Source: CAD feature listing. Evaluate the final solid. Frame: model axes, mm. A direction names the side the tool comes from. Give positions to 0.01 mm unless a question says otherwise; leave off trailing zeros. Write each loop counter-clockwise with the first axis right and the second up, starting at its lowest first coordinate (ties: lowest second). Pieces come first, ordered by that corner, then holes. Notation, with made-up numbers: (2, 45.5) -> (29, 45.5) arc R5 ccw to (29, 52.5) -> close; hole circle Ø6 at (-40, 72.25). An arc over 180 degrees is marked (long way). Use a Markdown table: item, result. Add a question column.
```python
from build123d import *

# Parameters (mm, degrees)
F0_W      = 29
F0_H      = 16.5
F1_DEPTH  = 38.5
F2_T      = -2
F3_DEPTH  = 2.25
F4_SIZE   = 2
F5_SIZE   = 0.99999
F7_DEPTH  = 16.501
F9_DEPTH  = 2
F10_R     = 2
F11_DEPTH = 2.001
F12_W     = 5.538
F12_H     = 5.533
F14_W     = 5.538
F14_H     = 4.583


# Not quite as in the source:
# - a fillet or chamfer is up to 0.001 mm smaller than in the source, because OpenCascade refuses the exact size


with BuildPart() as f1:
    # F0 (on Top) → F1 (new body)
    with BuildSketch(Plane.XY):
        with Locations((14.5, 8.25)):
            Rectangle(F0_W, F0_H)
    extrude(amount=F1_DEPTH)

    # F2
    f2_openings = [f1.faces().sort_by_distance(p)[0] for p in [
        (14.5, 8.25, 38.5),
    ]]
    offset(amount=F2_T, openings=f2_openings)

    # F3 (add): a face of the model
    f3_faces = [f1.faces().sort_by_distance(p)[0] for p in [
        (14.5, 8.25, 2),
    ]]
    extrude(f3_faces, amount=F3_DEPTH)

    # F4
    f4_edges = [f1.edges().sort_by_distance(p)[0] for p in [
        (29, 0, 19.25),
        (29, 16.5, 19.25),
        (0, 0, 19.25),
        (0, 16.5, 19.25),
        (14.5, 0, 0),
        (0, 8.25, 0),
        (14.5, 16.5, 0),
        (29, 8.25, 0),
    ]]
    chamfer(f4_edges, length=F4_SIZE)

    # F5 (size 1 in the source; OpenCascade refuses exactly that, so slightly less here)
    f5_edges = [f1.edges().sort_by_distance(p)[0] for p in [
        (14.5, 0, 38.5),
        (29, 8.25, 38.5),
        (14.5, 16.5, 38.5),
        (0, 8.25, 38.5),
    ]]
    chamfer(f5_edges, length=F5_SIZE)

    # F6 (on face) → F7 (cut, through all)
    with BuildSketch(Plane.XZ):
        Polygon((6.464, 8.664), (6.464, 4.94), (23.536, 4.94), (23.536, 8.664), (17.364, 12.834), (12.635, 12.834), align=None)
    extrude(amount=-F7_DEPTH, mode=Mode.SUBTRACT)

    # F8 (on Right) → F9 (cut, through all)
    with BuildSketch(Plane.YZ):
        with BuildLine():
            Line((14.5, 38.5), (2, 38.5))
            Line((2, 38.5), (2, 28.5))
            ThreePointArc((2, 28.5), (8.25, 34.75), (14.5, 28.5))
            Line((14.5, 28.5), (14.5, 38.5))
        make_face()
        with BuildLine():
            ThreePointArc((14.5, 28.5), (8.25, 34.75), (2, 28.5))
            Line((2, 28.5), (14.5, 28.5))
        make_face()
        with BuildLine():
            Line((14.5, 28.5), (2, 28.5))
            ThreePointArc((2, 28.5), (2.8042583777, 25.4330148055), (5.0100474186, 23.1553571429))
            ThreePointArc((5.0100474186, 23.1553571429), (8.25, 26.15), (11.4899525814, 23.1553571429))
            ThreePointArc((11.4899525814, 23.1553571429), (13.6957416223, 25.4330148055), (14.5, 28.5))
        make_face()
        with BuildLine():
            ThreePointArc((11.4899525814, 23.1553571429), (8.25, 26.15), (5.0100474186, 23.1553571429))
            ThreePointArc((5.0100474186, 23.1553571429), (8.25, 22.25), (11.4899525814, 23.1553571429))
        make_face()
        with BuildLine():
            ThreePointArc((11.4899525814, 23.1553571429), (8.25, 22.25), (5.0100474186, 23.1553571429))
            ThreePointArc((5.0100474186, 23.1553571429), (8.122222634, 19.6525128261), (11.5, 22.9))
            ThreePointArc((11.5, 22.9), (11.4974871739, 23.027777366), (11.4899525814, 23.1553571429))
        make_face()
    extrude(amount=F9_DEPTH, mode=Mode.SUBTRACT)

    # F10 (on face) → F11 (cut, through all)
    with BuildSketch(Plane(origin=(27, 0, 0), x_dir=(0, -1, 0), z_dir=(-1, 0, 0))):
        with Locations((-8.25, 22.9)):
            Circle(F10_R)
    extrude(amount=-F11_DEPTH, mode=Mode.SUBTRACT)

    # F12 (on face) → F15 section 0
    with BuildSketch(Plane(origin=(0, 0, 0), x_dir=(0, -1, 0), z_dir=(-1, 0, 0))):
        with Locations((-8.25, 8.0385)):
            Rectangle(F12_W, F12_H)
    # F14 (on offset) → F15 section 1
    with BuildSketch(Plane(origin=(4.45, 0, 0), x_dir=(0, -1, 0), z_dir=(-1, 0, 0))):
        with Locations((-8.25, 8.5135)):
            Rectangle(F14_W, F14_H)
    loft(mode=Mode.SUBTRACT)


solid = f1.part
```
(1) Access query for faces 1 (the flat face through (15, 15, 4.94)), 2 (the flat face through (2, 8, 14)), 3 (the flat face through (1.4, 1.4, 1.2)), 4 (the flat face through (1, 8, 10.805)). Directions: +Z, -Z, +X, -X, +Y, -Y. A direction counts if a zero-diameter tool reaches every point of the face in a straight line with its end or side. Return the directions, or none.
(2) Mould query, pull axis Y, two halves, no side actions, for faces 5 (the flat face through (20.49, 0.99, 10.72)), 6 (the flat face through (14, 8, 4.25)), 7 (the flat face through (14, 16, 38)), 8 (the flat face through (14, 1, 1)). Classes: +Y half, -Y half, draft (parallel to the pull), parting line (faces both ways), or undercut.
(3) First-contact query: pin 1 Ø1.5 at (x, y) = (21.5, 12.5) entering from +Z; pin 2 Ø1 at (y, z) = (1, 6.5) entering from +X; pin 3 Ø0.6 at (x, y) = (0.5, 7) entering from -Z. Flat tips, straight axial feed; report the tip coordinate or a pass-through.
(4) Cut plane A-A on x = 16. Return the cut outline in (y, z).
(5) Cut plane C-C on y = 13.25. Return the cut outline in (x, z).
(6) Material intervals for L1, parallel to Y at x = 25, z = 9; L2, parallel to X at y = 12.25, z = 4.5; L3, parallel to Z at x = 17, y = 14, sorted ascending.
(7) Cut plane B-B on z = 16. Return the cut outline in (x, y).
(8) Cut plane D-D on y = 8.25. Return the cut outline in (x, z) (3 decimals).
Output:
| question | item | result |
|---|---|---|
| 1 | face 1 | +Y, -Y |
| 1 | face 2 | +Z |
| 1 | face 3 | -Z, -X, -Y |
| 1 | face 4 | -X |
| 2 | face 5 | draft |
| 2 | face 6 | undercut |
| 2 | face 7 | +Y half |
| 2 | face 8 | -Y half |
| 3 | pin 1 | z = 4.25 |
| 3 | pin 2 | x = 28.5 |
| 3 | pin 3 | z = 1.2 |
| 4 | outline | (0, 2) -> (2, 0) -> (14.5, 0) -> (16.5, 2) -> (16.5, 4.94) -> (14.5, 4.94) -> (14.5, 4.25) -> (2, 4.25) -> (2, 4.94) -> (0, 4.94) -> close; (0, 12.83) -> (2, 12.83) -> (2, 38.5) -> (1, 38.5) -> (0, 37.5) -> close; (14.5, 12.83) -> (16.5, 12.83) -> (16.5, 37.5) -> (15.5, 38.5) -> (14.5, 38.5) -> close |
| 5 | outline | (0, 2) -> (2, 0) -> (27, 0) -> (29, 2) -> (29, 37.5) -> (28, 38.5) -> (27, 38.5) -> (27, 4.25) -> (2, 4.25) -> (2, 24.75) -> (0, 24.75) -> close |
| 6 | L1 | 0 to 2, 14.5 to 16.5 |
| 6 | L2 | 0 to 2, 27 to 29 |
| 6 | L3 | 0 to 4.25 |
| 7 | outline | (0, 2) -> (2, 0) -> (27, 0) -> (29, 2) -> (29, 14.5) -> (27, 16.5) -> (2, 16.5) -> (0, 14.5) -> close; hole (2, 2) -> (27, 2) -> (27, 14.5) -> (2, 14.5) -> close |
| 8 | outline | (0, 2) -> (2, 0) -> (27, 0) -> (29, 2) -> (29, 20.9) -> (27, 20.9) -> (27, 4.25) -> (2, 4.25) -> (2, 5.699) -> (0, 5.272) -> close; (0, 10.805) -> (2, 10.805) -> (2, 19.65) -> (0, 19.65) -> close; (27, 24.9) -> (29, 24.9) -> (29, 37.5) -> (28, 38.5) -> (27, 38.5) -> close |
